```python
from build123d import *

# Parameters (mm, degrees)
F1_DEPTH  = 12.7
F2_SIZE   = 19.05
F3_R      = 6.35
F3_R_2    = 7.9375
F4_DEPTH  = 25.4
F3_W      = 12.7
F3_H      = 120.65
F5_DEPTH  = 107.95
F6_SIZE   = 19.05
F8_DEPTH  = 193.548
F7_R      = 15.625598
F9_DEPTH  = 161.538807
F3_W_2    = 66.287807
F3_H_2    = 9.525
F10_DEPTH = 76.2
F12_DEPTH = 57.151


with BuildPart() as f1:
    # F0 (on Front) → F1 (new body)
    with BuildSketch(Plane.XZ):
        Polygon((103.08338, 64.568961), (-58.454427, 64.568961), (-119.16662, -17.981039), (-119.16662, -56.081039), (103.08338, -56.081039), align=None)
    extrude(amount=F1_DEPTH)

    # F2
    f2_edges = [f1.edges().sort_by_distance(p)[0] for p in [
        (103.08338, -6.35, -56.081039),
        (103.08338, -6.35, 64.568961),
    ]]
    chamfer(f2_edges, length=F2_SIZE)

    # F3 (on face) → F4 (cut)
    with BuildSketch(Plane.XZ.offset(12.7)):
        with Locations((78.070573, -37.031039)):
            Circle(F3_R)
        with Locations((78.070573, 39.168961)):
            Circle(F3_R)
        with Locations((-2.419149, 32.818961)):
            Circle(F3_R_2)
        with Locations((-10.829427, -43.381039)):
            Circle(F3_R_2)
        with Locations((-106.079427, -43.381039)):
            Circle(F3_R)
    extrude(amount=-F4_DEPTH, mode=Mode.SUBTRACT)

    # F3 (on face) → F5 (join)
    with BuildSketch(Plane.XZ.offset(12.7)):
        with Locations((-52.104427, 4.243961)):
            Rectangle(F3_W, F3_H)
        Polygon((36.795573, 64.568961), (24.095573, 64.568961), (24.095573, -56.081039), (36.795573, -56.081039), (36.795573, -8.456039), (36.795573, 1.068961), align=None)
    extrude(amount=F5_DEPTH)

    # F6
    f6_edges = [f1.edges().sort_by_distance(p)[0] for p in [
        (-52.104427, -120.65, -56.081039),
        (30.445573, -120.65, -56.081039),
    ]]
    chamfer(f6_edges, length=F6_SIZE)

    # F7 (on face) → F8 (cut)
    with BuildSketch(Plane(origin=(-58.454427, 0, 0), x_dir=(0, -1, 0), z_dir=(-1, 0, 0))):
        Polygon((38.1, 64.568961), (120.65, 1.068961), (120.65, 64.568961), align=None)
    extrude(amount=-F8_DEPTH, mode=Mode.SUBTRACT)

    # F7 (on face) → F9 (cut, through all)
    with BuildSketch(Plane(origin=(-58.454427, 0, 0), x_dir=(0, -1, 0), z_dir=(-1, 0, 0))):
        with Locations((82.55, -17.981039)):
            Circle(F7_R)
    extrude(amount=-F9_DEPTH, mode=Mode.SUBTRACT)

    # F3 (on face) → F10 (join)
    with BuildSketch(Plane.XZ.offset(12.7)):
        with Locations((69.939476, -3.693539)):
            Rectangle(F3_W_2, F3_H_2)
    extrude(amount=F10_DEPTH)

    # F11 (on face) → F12 (cut, through all)
    with BuildSketch(Plane.XY.offset(1.068961)):
        Polygon((103.08338, -25.4), (49.495573, -88.9), (103.08338, -88.9), align=None)
    extrude(amount=-F12_DEPTH, mode=Mode.SUBTRACT)


solid = f1.part
```
CAD build for the part. Positions are in the model's coordinates, mm. A direction names the side the tool comes from. Round coordinates to 2 decimals unless told otherwise and drop trailing zeros. Loops run counter-clockwise (first coordinate to the right, second up) from the corner with the lowest first, then second, coordinate; pieces in that order, holes last. Notation, with made-up numbers: (-38, 15) - (-5, 15) arc R32 ccw to (-5, 49) - close; hole circle Ø7 at (-27, 84.5). An arc over 180 degrees is marked (long way). Return JSON: item names as keys, results as strings. Group by question number.
Q1. Drill centre lines: line 1 along X through (y, z) = (-55, 46.5); line 2 along Y through (x, z) = (46, -25.5); line 3 along Y through (x, z) = (-55.5, -14.5). Where is each one in solid material? Low to high. Write a range as [from, to].
Q2. Band-saw the part on C-C on y = -82.55. Give the cut face in (x, z).
Q3. Flat gauge pins, fed straight in: pin 1 Ø10 at (y, z) = (-77.5, -43) entering from -X; pin 2 Ø11.5 at (x, z) = (78.07, 39.17) entering from -Y; pin 3 Ø5 at (y, z) = (-79.5, -6.5) entering from -X; pin 4 Ø4 at (y, z) = (-45, -19.5) entering from +X. Where does each tip first touch, or does it go through?
Q4. Tool access for faces 4 (the face through (-52.19, -66.94, -17.29)), 5 (the face through (36.796, -54, -10)), 6 (the face through (62, -42, 1.069)): list every direction of +Z, -Z, +X, -X, +Y, -Y with a clear straight run to the whole face (end or side of a thin tool).
Q5. Two-plate mould, pull along X, no slides. Class faces 1 (the face through (-52.19, -111.26, -46.42)), 2 (the face through (103.083, -19, -4)), 3 (the face through (-100.214, -6.439, -45.813)): +X half, -X half, draft (parallel to the pull), parting line (faces both ways), or undercut.
Q6. Band-saw the part on D-D on x = -39.5. Give the cut face in (y, z), plus the area to 3 significant figures.
Q7. Band-saw the part on A-A on y = -34.5. Give the cut face in (x, z), plus the area to 3 significant figures.
Q8. Band-saw the part on B-B on z = 29.5. Give the cut face in (x, y), plus the area to 3 significant figures.
Solutions:
{
 "1": {"line 1": "x = [-58.45, -45.75], [24.1, 36.8]", "line 2": "y = [-12.7, 0]", "line 3": "y = [-120.65, -97.78], [-67.32, 0]"},
 "2": {"outline": "(-58.45, -56.08) - (-45.75, -56.08) - (-45.75, -33.61) - (-58.45, -33.61) - close; (-58.45, -2.36) - (-45.75, -2.36) - (-45.75, 30.38) - (-58.45, 30.38) - close; (24.1, -56.08) - (36.8, -56.08) - (36.8, -33.61) - (24.1, -33.61) - close; (24.1, -2.36) - (36.8, -2.36) - (36.8, -8.46) - (54.85, -8.46) - (54.85, 1.07) - (36.8, 1.07) - (36.8, 30.38) - (24.1, 30.38) - close"},
 "3": {"pin 1": "stops at x = -58.45", "pin 2": "passes through", "pin 3": "stops at x = 36.8", "pin 4": "stops at x = 36.8"},
 "4": {"face 4": "-X", "face 5": "+X, -Y", "face 6": "+Z, +X, -Y"},
 "5": {"face 1": "draft", "face 2": "+X half", "face 3": "undercut"},
 "6": {"outline": "(-12.7, -56.08) - (0, -56.08) - (0, 64.57) - (-12.7, 64.57) - close", "area": "1,530 mm^2"},
 "7": {"outline": "(-58.45, -56.08) - (-45.75, -56.08) - (-45.75, 64.57) - (-58.45, 64.57) - close; (24.1, -56.08) - (36.8, -56.08) - (36.8, -8.46) - (95.4, -8.46) - (95.4, 1.07) - (36.8, 1.07) - (36.8, 64.57) - (24.1, 64.57) - close", "area": "3,620 mm^2"},
 "8": {"outline": "(-84.25, -12.7) - (-58.45, -12.7) - (-58.45, -83.69) - (-45.75, -83.69) - (-45.75, -12.7) - (-9.63, -12.7) - (-9.63, 0) - (-84.25, 0) - close; (4.79, -12.7) - (24.1, -12.7) - (24.1, -83.69) - (36.8, -83.69) - (36.8, -12.7) - (103.08, -12.7) - (103.08, 0) - (4.79, 0) - close", "area": "4,000 mm^2"}
}
